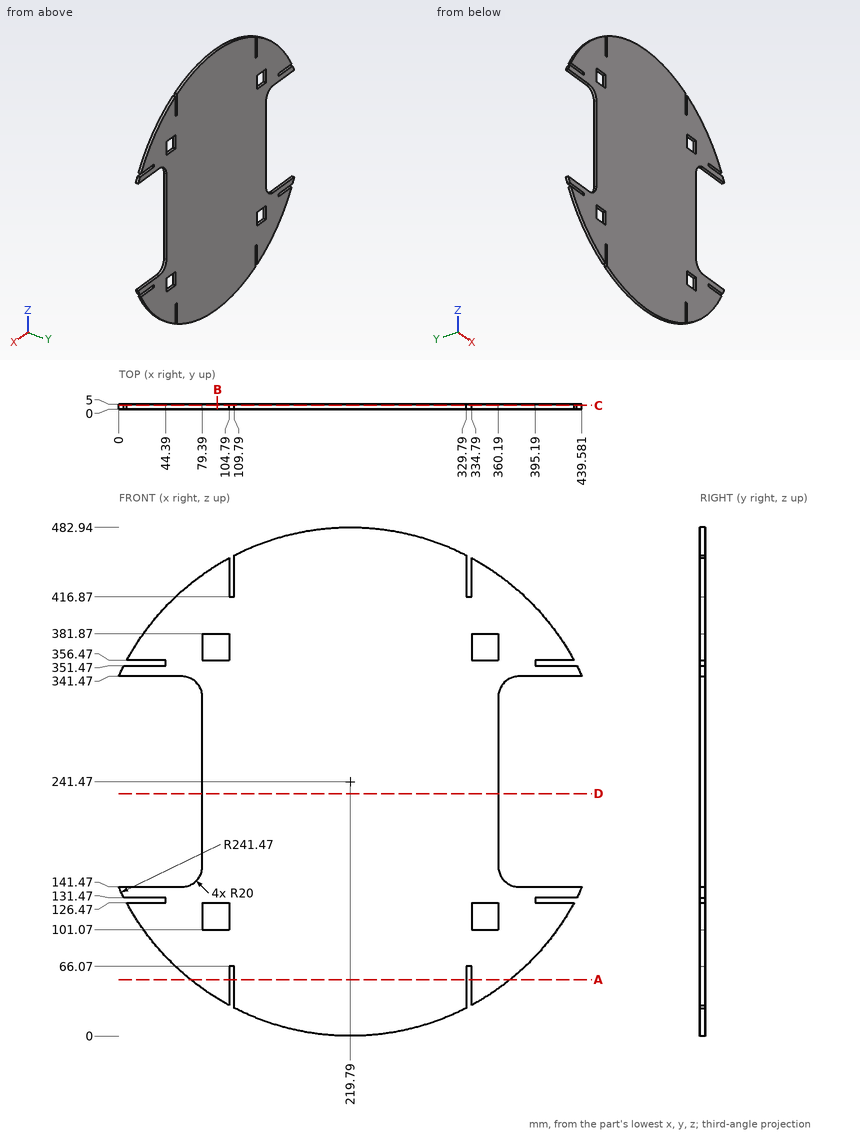
Check sheet for the drawn part. Datum: minimum x, y, z corner. Units: mm. Round coordinates to 2 decimals unless told otherwise and drop trailing zeros. Order: outer loops, then holes, each group sorted by start corner. A loop starts at its lowest first (then second) coordinate and runs counter-clockwise, first axis right, second up. Notation, with made-up numbers: (0.25, -11) -> (4.25, -11) arc R19 ccw to (4.25, -5) -> close; hole circle Ø6 at (-37.5, -14.5). An arc over 180 degrees is marked (long way). Put each result on its own line as item: value. Start each with the question number.
(1) Material ranges on line 1 along Z through (x, y) = (98.5, 1.1); line 2 along X through (y, z) = (0.6, 442.5) (1 decimal); line 3 along Z through (x, y) = (100, 3.75), recorded low to high.
(2) Section check A-A (z = 53.5). Enter the section's corners in (x, y) (1 decimal).
(3) Section check D-D (z = 230). Enter the section's corners in (x, y).
(4) Section check B-B (x = 93.5). Enter the section's corners in (y, z), then the cut area to 3 significant figures.
(5) Depth check by flat-ended pin: pin 1 Ø1 at (y, z) = (1.5, 381.5) entering from +X; pin 2 Ø3 at (y, z) = (1, 316) entering from -X; pin 3 Ø1.5 at (x, y) = (89, 2) entering from +Z. Enter the tip coordinate at first touch or a pass-through.
(6) Section check C-C (y = 3.7). State how many separate pieces and enclosed holes the cut face has, then the cut area to 3 significant figures.
Completed:
1. line 1: z = 32.67 to 101.07, 126.47 to 356.47, 381.87 to 450.27
1. line 2: x = 86 to 104.8, 109.8 to 329.8, 334.8 to 353.6
1. line 3: z = 31.81 to 101.07, 126.47 to 356.47, 381.87 to 451.13
2. outline: (68.2, 0) -> (104.8, 0) -> (104.8, 5) -> (68.2, 5) -> close; (109.8, 0) -> (329.8, 0) -> (329.8, 5) -> (109.8, 5) -> close; (334.8, 0) -> (371.4, 0) -> (371.4, 5) -> (334.8, 5) -> close
3. outline: (79.39, 0) -> (360.19, 0) -> (360.19, 5) -> (79.39, 5) -> close
4. outline: (0, 35.66) -> (5, 35.66) -> (5, 101.07) -> (0, 101.07) -> close; (0, 126.47) -> (5, 126.47) -> (5, 356.47) -> (0, 356.47) -> close; (0, 381.87) -> (5, 381.87) -> (5, 447.28) -> (0, 447.28) -> close
4. area: 1,800 mm2
5. pin 1: stops at x = 416.87
5. pin 2: stops at x = 79.39
5. pin 3: stops at z = 444.93
6. separate pieces: 1
6. enclosed holes: 4
6. area: 142,000 mm2
